Answer from the drawing. Dimensions are ordinates in mm from the lowest x, y and z of the part. A direction names the side the tool comes from. Coordinates: 2 decimals unless noted, no trailing zeros. Loops run counter-clockwise (first coordinate to the right, second up) from the corner with the lowest first, then second, coordinate; pieces in that order, holes last.
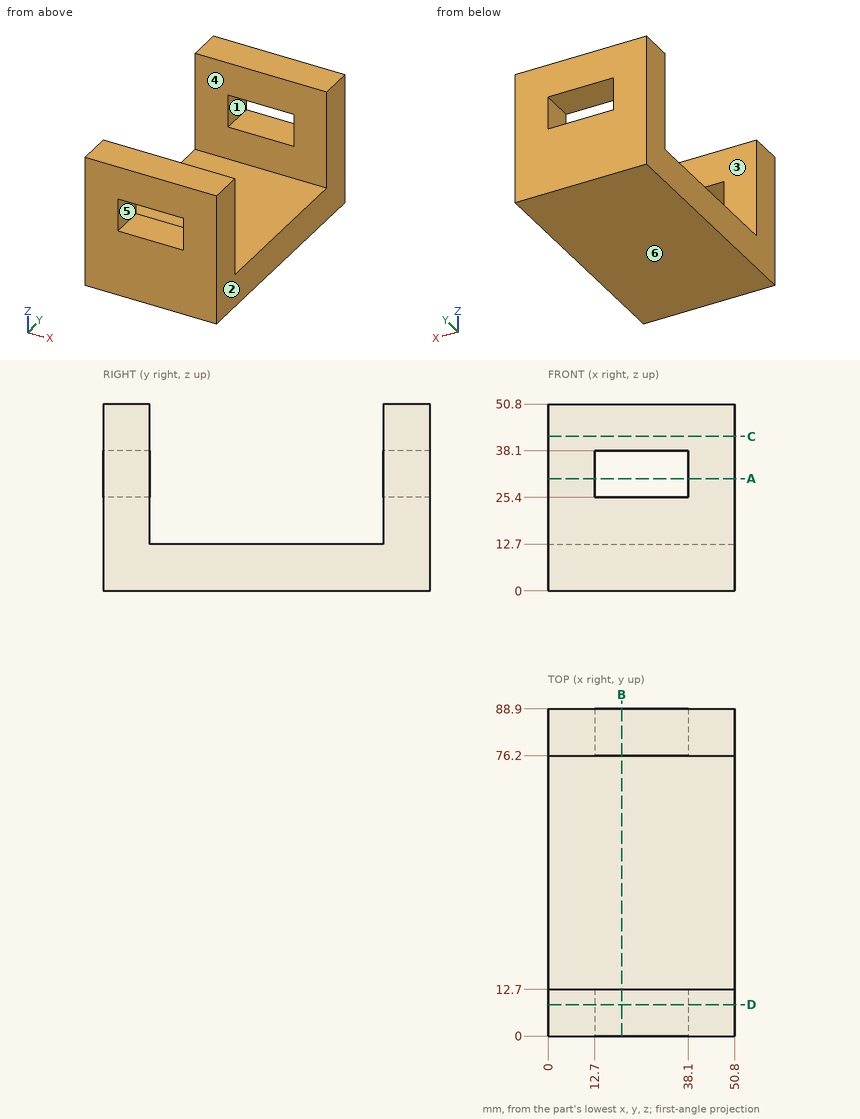
Item 1: Determine the mould class of the marked faces 4, 5 and 6 for opening direction Z: released by +Z, released by -Z, zero draft, split by the parting line, or undercut.
Numbers:
face 4: zero draft
face 5: undercut
face 6: released by -Z
Item 2: A cutting plane is placed at A-A on z = 30.5. Determine the outline of the cut face in (x, y), then the cut area to 3 significant figures.
Numbers:
outline: (0, 0) - (12.7, 0) - (12.7, 12.7) - (0, 12.7) - close; (0, 76.2) - (12.7, 76.2) - (12.7, 88.9) - (0, 88.9) - close; (38.1, 0) - (50.8, 0) - (50.8, 12.7) - (38.1, 12.7) - close; (38.1, 76.2) - (50.8, 76.2) - (50.8, 88.9) - (38.1, 88.9) - close
area: 645 mm2
Item 3: Find the intervals of material crossed by line 1 along Y through (x, z) = (45, 40.5); line 2 along Z through (x, y) = (22, 8); line 3 along Z through (x, y) = (35.5, 68.5), in increasing order.
Numbers:
line 1: y = 0 to 12.7, 76.2 to 88.9
line 2: z = 0 to 25.4, 38.1 to 50.8
line 3: z = 0 to 12.7
Item 4: A cutting plane is placed at C-C on z = 42. Determine the outline of the cut face in (x, y).
Numbers:
outline: (0, 0) - (50.8, 0) - (50.8, 12.7) - (0, 12.7) - close; (0, 76.2) - (50.8, 76.2) - (50.8, 88.9) - (0, 88.9) - close
Item 5: Which of the six approach directions +Z, -Z, +X, -X, +Y, -Y give full straight-line access (tool end or side, diameter ignored) to the marked faces 1, 2 and 3?
Numbers:
face 1: +Y, -Y
face 2: +Z, -Z, +X, +Y, -Y
face 3: +Z, +X, -X
Item 6: A cutting plane is placed at B-B on x = 20. Determine the outline of the cut face in (y, z).
Numbers:
outline: (0, 0) - (88.9, 0) - (88.9, 25.4) - (76.2, 25.4) - (76.2, 12.7) - (12.7, 12.7) - (12.7, 25.4) - (0, 25.4) - close; (0, 38.1) - (12.7, 38.1) - (12.7, 50.8) - (0, 50.8) - close; (76.2, 38.1) - (88.9, 38.1) - (88.9, 50.8) - (76.2, 50.8) - close
Item 7: A cutting plane is placed at D-D on y = 8.5. Determine the outline of the cut face in (x, z), then the cut area to 3 significant figures.
Numbers:
outline: (0, 0) - (50.8, 0) - (50.8, 50.8) - (0, 50.8) - close; hole (12.7, 25.4) - (38.1, 25.4) - (38.1, 38.1) - (12.7, 38.1) - close
area: 2,260 mm2
